from build123d import *

# Parameters (mm, degrees)
F0_W         = 15.8
F0_H         = 32
F1_DEPTH     = 3
F3_DEPTH     = 0.8
F5_W         = 4.6
F5_H         = 1.2
F6_DEPTH     = 2.4
F8_DEPTH     = 0.6
F9_W         = 4.6
F9_H         = 0.3
F10_DEPTH    = 0.4
F11_T1_DEPTH = 6.1
F12_SIZE2    = 1.49999
F12_SIZE     = 2.99999


# Not quite as in the source:
# - a fillet or chamfer that OpenCascade refuses, or shapes differently, is made with other operations: its cross-section is extruded or revolved along the edge and cut away or added
# - a fillet or chamfer is up to 0.001 mm smaller than in the source, because OpenCascade refuses the exact size


with BuildPart() as f1:
    # F0 (on Top) → F1 (new body)
    with BuildSketch(Plane.XY):
        with Locations((0, -4.9953348935)):
            Rectangle(F0_W, F0_H)
    extrude(amount=F1_DEPTH)

    # F2 (on face) → F3 (join)
    with BuildSketch(Plane.YZ.offset(7.9)):
        Polygon((11.0046651065, 0), (11.0046651065, 3), (5.5046651065, 3), (5.5046651065, 1.2), (3.0046651065, 1.2), (3.0046651065, 0), align=None)
    extrude(amount=F3_DEPTH)

    # F4: F1 across plane


with BuildPart() as f1_1:
    add(f1.part)
    add(f1.part.mirror(Plane.YZ))

    # F5 (on face) → F6 (join)
    with BuildSketch(Plane.XZ.offset(20.9953348935)):
        with Locations((0, 0.6)):
            Rectangle(F5_W, F5_H)
    extrude(amount=F6_DEPTH)

    # F7 (on face) → F8 (cut)
    with BuildSketch(Plane.XY.offset(3)):
        with BuildLine():
            Line((4, 7.3774643242), (-4, 7.3774643242))
            ThreePointArc((-4, 7.3774643242), (0, 3.5808500116), (4, 7.3774643242))
        make_face()
    extrude(amount=-F8_DEPTH, mode=Mode.SUBTRACT)

    # F9 (on face) → F10 (join)
    with BuildSketch(Plane.XY.offset(1.2)):
        with Locations((0, -23.2453348935)):
            Rectangle(F9_W, F9_H)
    extrude(amount=F10_DEPTH)

    # F11: fillet of radius 0.3 on 2 edges, made by hand

    # F11_s2 → F11_t1 (cut)
    with BuildSketch(Plane.YZ.offset(-3.05)):
        with BuildLine():
            ThreePointArc((-23.0953348935, 1.6), (-23.3074669278, 1.5121320344), (-23.3953348935, 1.3))
            Line((-23.3953348935, 1.3), (-23.3953348935, 1.6))
            Line((-23.3953348935, 1.6), (-23.0953348935, 1.6))
        make_face()
        with BuildLine():
            ThreePointArc((-23.0953348935, 1.3), (-23.1832028591, 1.5121320344), (-23.3953348935, 1.6))
            Line((-23.3953348935, 1.6), (-23.0953348935, 1.6))
            Line((-23.0953348935, 1.6), (-23.0953348935, 1.3))
        make_face()
    extrude(amount=F11_T1_DEPTH, mode=Mode.SUBTRACT)

    # F12 (size 3 and 1.5 in the source; OpenCascade refuses exactly that, so slightly less here)
    f12_edges = [f1_1.edges().sort_by_distance(p)[0] for p in [
        (0, 11.004665, 3),
    ]]
    chamfer(f12_edges, length=F12_SIZE, length2=F12_SIZE2)


solid = f1_1.part
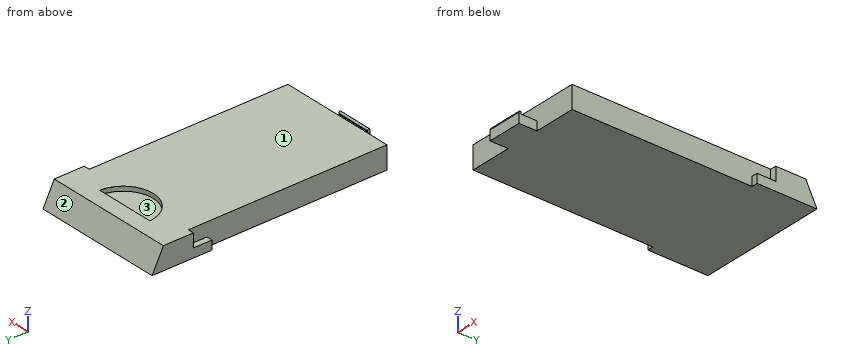
Geometry check sheet. Reference: the model listing, model coordinates, mm. Face numbers are marked on the shaded views. Give positions to 0.01 mm unless a question says otherwise; leave off trailing zeros. Order: outer loops, then holes, each group sorted by start corner. A loop starts at its lowest first (then second) coordinate and runs counter-clockwise, first axis right, second up. Notation, with made-up numbers: (37, -23) - (54, -23) arc R16 cw to (54, 0) - close; hole circle Ø11 at (-4, -34). An arc over 180 degrees is marked (long way). Use one line per item in the form item = value.
1) Draft check along Y on the marked faces 1, 2 and 3. Enter one of: released by +Y, released by -Y, zero draft, split by the parting line, or undercut.
Working result:
face_1 = zero draft
face_2 = released by +Y
face_3 = undercut
2) Depth check by flat-ended pin: pin 1 Ø0.9 at (x, z) = (-8.5, 1.5) entering from -Y; pin 2 Ø1.1 at (x, y) = (0, 4.5) entering from +Z; pin 3 Ø0.5 at (x, z) = (-1, 3) entering from -Y. Enter the tip coordinate at first touch or a pass-through.
Working result:
pin_1 = 3
pin_2 = 2.4
pin_3 = -21
3) Material ranges on probe 1 along X at (y, z) = (-6, 1.25); probe 2 along Y at (x, z) = (-5, 1.4); probe 3 along Y at (x, z) = (-1, 2.95), recorded low to high. Write a range as from..to.
Working result:
probe_1 = -7.9..7.9
probe_2 = -21..10.3
probe_3 = -21..3.71, 7.38..9.53
4) Sectioned sample at B-B (y = -20). Record the boundary of the cut face in (x, z), and give its area (3 significant figures).
Working result:
outline = (-7.9, 0) - (7.9, 0) - (7.9, 3) - (-7.9, 3) - close
area = 47.4 mm^2
5) Sectioned sample at C-C (z = 2). Record the boundary of the cut face in (x, y), and give its area (3 significant figures).
Working result:
outline = (-8.7, 5.5) - (-7.9, 5.5) - (-7.9, -21) - (7.9, -21) - (7.9, 5.5) - (8.7, 5.5) - (8.7, 10) - (-8.7, 10) - close
area = 497 mm^2
